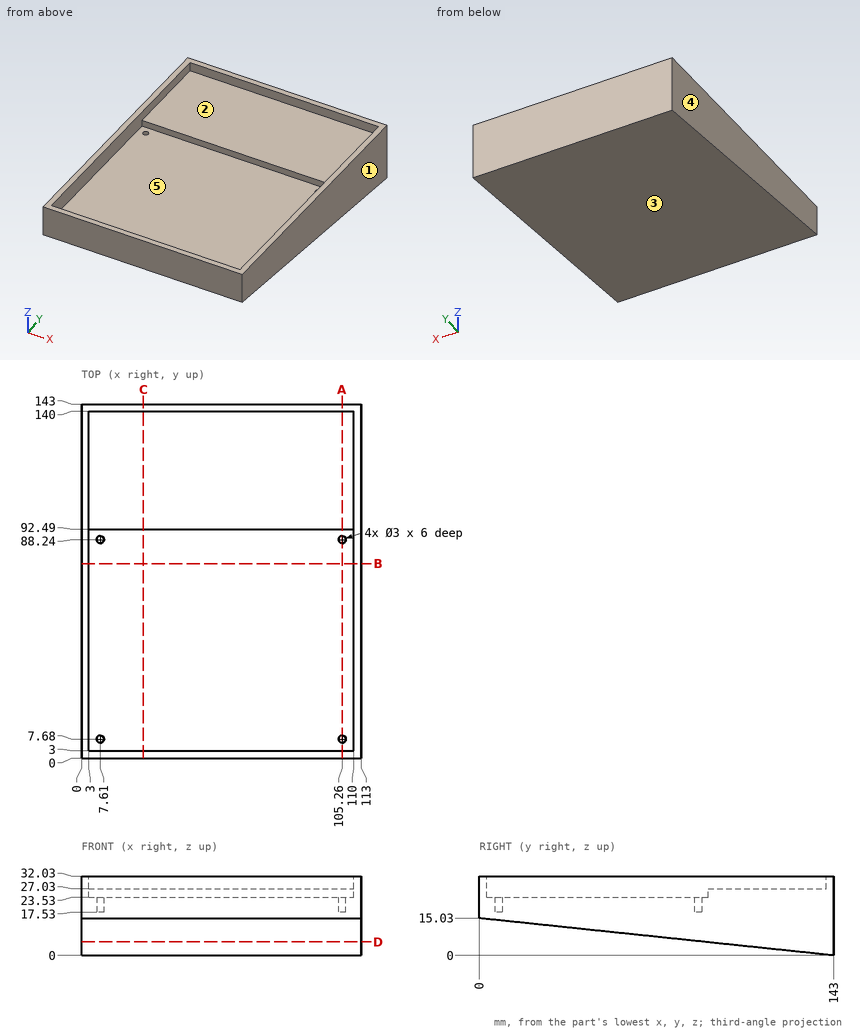
Source: three-view drawing plus pictorial views. Frame: mm from the lowest corner of the part. A direction names the side the tool comes from. Round coordinates to 2 decimals unless told otherwise and drop trailing zeros. Loops run counter-clockwise (first coordinate to the right, second up) from the corner with the lowest first, then second, coordinate; pieces in that order, holes last.
Q1. First-contact query: P1, Ø1.8, axis at x = 7.61, y = 7.68, coming from the +Z side; P2, Ø1.8, axis at x = 7.61, y = 88.24, coming from the -Z side; P3, Ø2.5, axis at x = 105.26, y = 88.24, coming from the -Z side. Flat tips, straight axial feed; report the tip coordinate or a pass-through.
Q2. Section B-B, the plane y = 78.5. Return loops of the section in (x, z), plus the area to 3 significant figures.
Q3. Section A-A, the plane x = 105.26. Return loops of the section in (y, z).
Q4. Ray query, line 1 (Y direction, x = 105, z = 19); line 2 (X direction, y = 88, z = 21); line 3 (Y direction, x = 78, z = 24). Return the intervals inside material, ascending.
Q5. Mould query, pull axis Y, two halves, no side actions, for the marked faces 1, 2 and 3. Classes: pulls with the +Y half, pulls with the -Y half, needs draft (parallel to the pull), parting line crosses it, or undercut.
Q6. Access query for the marked faces 4 and 5. Directions: +Z, -Z, +X, -X, +Y, -Y. A direction counts if a zero-diameter tool reaches every point of the face in a straight line with its end or side. Return the directions, or none.
Q7. Section C-C, the plane x = 25. Return loops of the section in (y, z), plus the area to 3 significant figures.
Q8. Section D-D, the plane z = 5.5. Return loops of the section in (x, y).
Solutions:
1. P1: stops at z = 17.53
1. P2: stops at z = 5.66
1. P3: stops at z = 5.62
2. outline: (0, 6.78) - (113, 6.78) - (113, 32.03) - (110, 32.03) - (110, 23.53) - (3, 23.53) - (3, 32.03) - (0, 32.03) - close
2. area: 1,940 mm2
3. outline: (0, 15.03) - (143, 0) - (143, 32.03) - (140, 32.03) - (140, 27.03) - (92.49, 27.03) - (92.49, 23.53) - (89.74, 23.53) - (89.74, 17.53) - (86.74, 17.53) - (86.74, 23.53) - (9.18, 23.53) - (9.18, 17.53) - (6.18, 17.53) - (6.18, 23.53) - (3, 23.53) - (3, 32.03) - (0, 32.03) - close
4. line 1: y = 0 to 6.2, 9.16 to 86.76, 89.72 to 143
4. line 2: x = 0 to 6.13, 9.09 to 103.78, 106.74 to 113
4. line 3: y = 0 to 3, 92.49 to 143
5. face 1: needs draft
5. face 2: undercut
5. face 3: pulls with the -Y half
6. face 4: +Z, -Z, -X, +Y, -Y
6. face 5: +Z
7. outline: (0, 15.03) - (143, 0) - (143, 32.03) - (140, 32.03) - (140, 27.03) - (92.49, 27.03) - (92.49, 23.53) - (3, 23.53) - (3, 32.03) - (0, 32.03) - close
7. area: 2,510 mm2
8. outline: (0, 90.67) - (113, 90.67) - (113, 143) - (0, 143) - close
